Read the model definition and answer for the solid it produces. Units are mm, in the model's axes. A direction names the side the tool comes from. Give positions to 0.01 mm unless a question says otherwise; leave off trailing zeros. Loops run counter-clockwise (first coordinate to the right, second up) from the corner with the lowest first, then second, coordinate; pieces in that order, holes last. Notation, with made-up numbers: (-4, 34.5) - (35, 34.5) arc R27 ccw to (35, 71.5) - close; hole circle Ø6 at (37, 86.25). An arc over 180 degrees is marked (long way). Write item = value, one per line.
Autodesk Inventor part; units mm, degrees
ref_plane "Plano de trabalho1" through (0, 30, 0) normal (0, 1, 0) x (-1, 0, 0)
ref_plane "Plano de trabalho5" through (0, 0, 16.148) normal (0, 0, 1) x (1, 0, 0)
ref_plane "YZ Plane" through (0, 0, 0) normal (1, 0, 0) x (0, 1, 0)
sketch "Esboço1" plane through (0, 0, 0) normal (0, 1, 0) x (-1, 0, 0)
  circle A0 centre (0, 0) radius 19
  circle A1 centre (0, 0) radius 14
  dimension "d0" = 38
  dimension "d1" = 28
extrude "Extrusão1" add sketch "Esboço1" along normal blind 30
sketch "Esboço2" plane through (0, 0, 0) normal (1, 0, 0) x (0, 1, 0)
  line L0 (-5, 5) -> (5, 5)
  line L1 (5, 5) -> (5, -5)
  line L2 (5, -5) -> (-5, -5)
  line L3 (-5, -5) -> (-5, 5)
  line L4 (-5, 5) -> (5, -5) construction
  line L5 (5, 5) -> (-5, -5) construction
  point P0 (0, 0)
  dimension "d4" = 10
  dimension "d5" = 10
extrude "Extrusão2" cut sketch "Esboço2" along normal mid plane 40
sketch "Esboço3" plane through (0, 0, 0) normal (0, 0, 1) x (1, 0, 0)
  point P0 (0, 0)
ref_plane "Plano de trabalho1" through (0, 30, 0) normal (0, 1, 0) x (-1, 0, 0)
sketch "Esboço4" plane through (0, 30, 0) normal (0, 1, 0) x (-1, 0, 0)
  circle A0 centre (0, 0) radius 19
  line L0 (10.0122, 16.148) -> (-10.0122, -16.148) construction
  line L1 (-10.0122, 16.148) -> (10.0122, -16.148) construction
  circle A1 centre (0, 0) radius 14
  line L2 (7.3774, 11.8985) -> (-7.3774, -11.8985) construction
  line L3 (-7.3774, 11.8985) -> (7.3774, -11.8985) construction
  line L4 (10.0122, -16.148) -> (7.3774, -11.8985)
  line L5 (-10.0122, -16.148) -> (-7.3774, -11.8985)
  line L6 (-10.0122, 16.148) -> (-7.3774, 11.8985)
  line L7 (7.3774, 11.8985) -> (10.0122, 16.148)
  arc A2 (-10.0122, -16.148) -> (10.0122, -16.148) centre (0, 0) ccw
  arc A3 (10.0122, 16.148) -> (-10.0122, 16.148) centre (0, 0) ccw
  arc A4 (7.3774, 11.8985) -> (-7.3774, 11.8985) centre (0, 0) ccw
  arc A5 (-7.3774, -11.8985) -> (7.3774, -11.8985) centre (0, 0) ccw
extrude "Extrusão3" cut sketch "Esboço4" against normal blind 19.3 contours L7 A1 L6 A0 | A0 L5 A1 L4
sketch "Esboço5" plane through (0, 30, 0) normal (0, 1, 0) x (-1, 0, 0)
  point P0 (0, 0)
ref_plane "Plano de trabalho4" through (0, 0, 19) normal (0, 0, 1) x (1, 0, 0)
sketch "Esboço6" plane through (0, 0, 19) normal (0, 0, 1) x (1, 0, 0)
  line L0 (-10.0122, 10.7) -> (-7.3774, 10.7)
  line L1 (7.3774, 10.7) -> (10.0122, 10.7)
  line L2 (13.0767, 0) -> (-13.0767, 0)
  line L3 (10.0122, 0) -> (-10.0122, 0)
  line L4 (-10.0122, 0) -> (10.0122, 0)
  line L5 (10.0122, 0) -> (10.0122, 5)
  line L6 (10.0122, 5) -> (-10.0122, 5)
  line L7 (-10.0122, 5) -> (-10.0122, 0)
  point P0 (0, 0)
  dimension "d20" = 5
extrude "Extrusão4" add sketch "Esboço6" along normal blind 20.048 and the other way blind 3
fillet "Arredondamento1" radius 3 2 edges at (-10.0122, 2.5, 39.048) (10.0122, 2.5, 39.048)
sketch "Esboço7" plane through (0, 0, 0) normal (1, 0, 0) x (0, 1, 0)
  line L0 (10.7, 16.148) -> (10.7, 11.8985)
  line L1 (5, 36.048) -> (5, 16.148)
  line L2 (10.7, 16.148) -> (5, 16.148)
  line L3 (5, 16.148) -> (5, 23.848)
  line L4 (5, 23.848) -> (10.7, 23.848)
  line L5 (10.7, 23.848) -> (10.7, 16.148)
  point P0 (0, 0)
  dimension "d28" = 7.7
extrude "Extrusão5" add sketch "Esboço7" along normal mid plane 20
chamfer "Chanfro1" distance 5.7 distance2 7.7 1 edges at (0, 10.7, 23.848) measured on face at (-3.3333, 6.9, 23.848)
sketch "Esboço8" plane through (-7.0122, 5, 39.048) normal (0, 1, 0) x (1, 0, 0)
  line L0 (0, 0) -> (14.0243, 0)
  line L1 (1.9995, 0) -> (1.9995, 7.85) construction
  line L2 (5.3995, 7.85) -> (3.6995, 4.9055)
  line L3 (3.6995, 4.9055) -> (0.2995, 4.9055)
  line L4 (0.2995, 4.9055) -> (-1.4005, 7.85)
  line L5 (-1.4005, 7.85) -> (0.2995, 10.7945)
  line L6 (0.2995, 10.7945) -> (3.6995, 10.7945)
  line L7 (3.6995, 10.7945) -> (5.3995, 7.85)
  line L8 (5.3995, 7.85) -> (8.5995, 7.85) construction
  line L9 (11.9995, 0) -> (11.9995, 7.85) construction
  line L10 (15.3995, 7.85) -> (13.6995, 4.9055)
  line L11 (13.6995, 4.9055) -> (10.2995, 4.9055)
  line L12 (10.2995, 4.9055) -> (8.5995, 7.85)
  line L13 (8.5995, 7.85) -> (10.2995, 10.7945)
  line L14 (10.2995, 10.7945) -> (13.6995, 10.7945)
  line L15 (13.6995, 10.7945) -> (15.3995, 7.85)
  line L16 (-1.4005, 7.85) -> (-3.0005, 7.85) construction
  line L17 (15.3995, 7.85) -> (16.9995, 7.85) construction
  line L18 (17.0243, 3) -> (17.0243, 22.9)
  line L19 (-3, 3) -> (-3, 22.9)
  line L20 (-3, 22.9) -> (-3, 3)
  point P0 (7.0122, 39.048)
  point P1 (-3, 7.85)
  dimension "d37" = 7.85
  dimension "d38" = 3.4
  dimension "d39" = 3.2
  dimension "d40" = 7.85
  dimension "d41" = 3.4
  dimension "d43" = 16.8
  dimension "d44" = 1.6
  dimension "d45" = 1.6
ref_plane "Plano de trabalho5" through (0, 0, 16.148) normal (0, 0, 1) x (1, 0, 0)
extrude "Extrusão6" cut sketch "Esboço8" against normal blind 3
sketch "Esboço9" plane through (-7.0122, 2, 39.048) normal (0, 1, 0) x (1, 0, 0)
  line L0 (0.2995, 10.7945) -> (3.6995, 10.7945) construction
  line L1 (5.3995, 7.85) -> (3.6995, 4.9055)
  line L2 (3.6995, 10.7945) -> (5.3995, 7.85)
  line L3 (0.2995, 10.7945) -> (3.6995, 10.7945)
  line L4 (-1.4005, 7.85) -> (0.2995, 10.7945)
  line L5 (0.2995, 4.9055) -> (-1.4005, 7.85)
  line L6 (3.6995, 4.9055) -> (0.2995, 4.9055)
  line L7 (3.6995, 10.7945) -> (0.2995, 4.9055) construction
  line L8 (0.2995, 10.7945) -> (3.6995, 4.9055) construction
  circle A0 centre (1.9995, 7.85) radius 1.8
  line L9 (15.3995, 7.85) -> (13.6995, 4.9055) construction
  line L10 (13.6995, 10.7945) -> (15.3995, 7.85) construction
  line L11 (10.2995, 10.7945) -> (13.6995, 10.7945) construction
  line L12 (8.5995, 7.85) -> (10.2995, 10.7945) construction
  line L13 (10.2995, 4.9055) -> (8.5995, 7.85) construction
  line L14 (13.6995, 4.9055) -> (10.2995, 4.9055) construction
  line L15 (13.6995, 10.7945) -> (10.2995, 4.9055) construction
  line L16 (10.2995, 10.7945) -> (13.6995, 4.9055) construction
  circle A1 centre (11.9995, 7.85) radius 1.8
  point P0 (7.0122, 39.048)
  dimension "d49" = 3.6
  dimension "d50" = 3.6
extrude "Extrusão7" cut sketch "Esboço9" against normal up to next contours A0 | A1
mirror "Espelhamento1" about plane through (0, 0, 0) normal (0, 0, 1) of "Extrusão4", "Arredondamento1", "Extrusão5", "Chanfro1", "Extrusão6", "Extrusão7"
sketch "Esboço11" plane through (-10, 5, -16.1555) normal (-1, 0, 0) x (0, 0, 1)
  line L0 (0, 5.6944) -> (-7.6925, 0)
  line L1 (0, 5.7) -> (-7.6925, 5.7)
  line L2 (-7.6925, 5.7) -> (-7.6925, 0)
  line L3 (-7.6925, 0) -> (0, 5.7)
  point P0 (16.1555, -5)
  point P1 (0, 0)
extrude "Extrusão9" cut sketch "Esboço11" against normal blind 20
sketch "Esboço12" plane through (0, 0, 0) normal (0, -1, 0) x (1, 0, 0)
  circle A0 centre (-5.0126, 31.198) radius 1.8
  circle A1 centre (4.9874, 31.198) radius 1.8
  circle A2 centre (4.9874, -31.198) radius 1.8
  circle A3 centre (-5.0126, -31.198) radius 1.8
  point P0 (0, 0)
properties part number "SuporteMotor"
1) A cutting plane is placed at A-A on z = 0. Determine the outline of the cut face in (x, y), then the cut area to 3 significant figures.
Output:
outline = (-19, 5) - (-14, 5) - (-14, 30) - (-19, 30) - close; (14, 5) - (19, 5) - (19, 30) - (14, 30) - close
area = 250 mm²
2) Find the intervals of material crossed by probe 1 along X at (y, z) = (15.25, 0); probe 2 along Z at (x, y) = (-12, 27.5); probe 3 along Y at (x, z) = (7, -33.5), in increasing order.
Output:
probe_1 = -19 to -14, 14 to 19
probe_2 = -14.73 to -7.21, 7.21 to 14.73
probe_3 = 0 to 2
3) A cutting plane is placed at C-C on y = 17.5. Determine the outline of the cut face in (x, z), then the cut area to 3 significant figures.
Output:
outline = (-10.01, -16.15) - (-7.38, -11.9) arc R14 cw to (-7.38, 11.9) - (-10.01, 16.15) arc R19 ccw to start; (7.38, -11.9) - (10.01, -16.15) arc R19 ccw to (10.01, 16.15) - (7.38, 11.9) arc R14 cw to start
area = 335 mm²
4) Each of these flat-tipped pins is pushed along its axis until it touches: P1, Ø6.5, axis at x = 17, z = 0, coming from the -Y side; P2, Ø2.5, axis at x = 15, y = 3, coming from the -Z side; P3, Ø3, axis at y = 7.5, z = 19, coming from the +X side; P4, Ø1.8, axis at x = -5, z = -30.5, coming from the +Y side. Where does it stop, or does it pass through?
Output:
P1 = 5
P2 = -13.11
P3 = 10
P4 = through
5) The mould has two halves that part along X. Classify faces 1 (the face through (0, 5, -33)), 2 (the face through (-5.403, 1.014, 32.955)), 3 (the face through (-10.012, 2, -26)): pulls with the +X half, pulls with the -X half, needs draft (parallel to the pull), parting line crosses it, or undercut.
Output:
face_1 = needs draft
face_2 = undercut
face_3 = pulls with the -X half
6) A tool of negligible diameter and unlimited length cuts with its end or side. For faces 4 (the face through (4.597, 1.014, 32.955)), 5 (the face through (8.71, 20.49, -14.05)), 6 (the face through (-7.55, 3.52, 32.69)), from which of +Z, -Z, +X, -X, +Y, -Y can it reach the whole face along a straight path? Write none if from no direction.
Output:
face_4 = +Y, -Y
face_5 = -Z, +Y
face_6 = +Y
